```python
from build123d import *

# Parameters (mm, degrees)
EXTRU_MINCE1_DEPTH      = 38.1
ESQUISSE2_R             = 1.89865
ENL_V_MAT_EXTRU_1_DEPTH = 228.663979486
ENL_V_MAT_EXTRU_2_DEPTH = 3.048
D_GAGEMENT_61_D         = 3.7973


with BuildPart() as part:
    # Esquisse1 → Extru.-Mince1 (new body)
    with BuildSketch(Plane.XY):
        Polygon((90.805, 44.088736397), (116.205, 44.088736397), (116.205, -223.011474044), (111.125, -223.011474044), (111.125, 39.008736397), (90.805, 39.008736397), align=None)
    extrude(amount=-EXTRU_MINCE1_DEPTH)

    # Esquisse2 → Enlèv. mat.-Extru.1 (cut, through all)
    with BuildSketch(Plane(origin=(116.205, 0, 0), x_dir=(0, 0, -1), z_dir=(1, 0, 0))):
        with Locations(Location((19.05, -202.469224044, 0), (0, 0, 90))):
            Circle(ESQUISSE2_R)
    extrude(amount=-ENL_V_MAT_EXTRU_1_DEPTH, mode=Mode.SUBTRACT)

    # Esquisse3 → Enlèv. mat.-Extru.2 (cut)
    with BuildSketch(Plane.XZ.offset(-39.008736397)):
        Polygon((100.965, -23.735650044), (96.774, -26.155325022), (96.774, -30.994674978), (100.965, -33.414349956), (105.156, -30.994674978), (105.156, -26.155325022), align=None)
        Polygon((100.965, -4.685650044), (96.774, -7.105325022), (96.774, -11.944674978), (100.965, -14.364349956), (105.156, -11.944674978), (105.156, -7.105325022), align=None)
    extrude(amount=-ENL_V_MAT_EXTRU_2_DEPTH, mode=Mode.SUBTRACT)

    # Dégagement #61 (through all)
    with Locations(Plane(origin=(0, 42.056736397, 0), x_dir=(-1, 0, 0), z_dir=(0, -1, 0))):
        with Locations((-100.965, 28.575), (-100.965, 9.525)):
            Hole(D_GAGEMENT_61_D / 2)


solid = part.part
```
Read the model definition and answer for the solid it produces. Units are mm, in the model's axes. A direction names the side the tool comes from. Give positions to 0.01 mm unless a question says otherwise; leave off trailing zeros. Order: outer loops, then holes, each group sorted by start corner. A loop starts at its lowest first (then second) coordinate and runs counter-clockwise, first axis right, second up.
(1) Given pin 1 (10 mm diameter, centred on x = 106, y = -130.5, fed in from -Z) (1 decimal); pin 2 (4 mm diameter, centred on x = 100, z = -28.5, fed in from -Y); pin 3 (6 mm diameter, centred on x = 97, z = -33, fed in from -Y), each flat-ended and moving along its own axis, determine where each tip first touches the part or whether it passes through.
(2) For faces 1 (the flat face through (101, 42.057, -12)), 2 (the flat face through (90.805, 42, -19)), 3 (the flat face through (111.125, -94, -19)), determine the directions among +Z, -Z, +X, -X, +Y, -Y from which every point of the face is accessible in a straight line to the end or side of a thin tool.
(3) Straight lines are drawn through the part: L1, parallel to X at y = 15, z = -9.5 (3 decimals); L2, parallel to Y at x = 99, z = -23; L3, parallel to Y at x = 112.5, z = -18. For each, find the intervals that lie inside material, in ascending order.
(4) For a pull along Z with two mould halves and no side action, classify faces 4 (the flat face through (101, 39.009, -19)), 5 (the flat face through (113, -69, 0)), 6 (the flat face through (101, 42.057, -31)) as released by +Z, released by -Z, zero draft, split by the parting line, or undercut.
(5) Find section A-A (y = -187). Give the vertices of the cut face in (x, z) (3 decimals).
Result sheet:
1. pin 1: passes through
1. pin 2: stops at y = 42.06
1. pin 3: stops at y = 39.01
2. face 1: -Y
2. face 2: +Z, -Z, -X, +Y, -Y
2. face 3: +Z, -Z, -X, -Y
3. L1: x = 111.125 to 116.205
3. L2: y = 39.01 to 44.09
3. L3: y = -223.01 to -204.05, -200.89 to 44.09
4. face 4: zero draft
4. face 5: released by +Z
4. face 6: undercut
5. outline: (111.125, -38.1) - (116.205, -38.1) - (116.205, 0) - (111.125, 0) - close
